```python
from build123d import *

# Parameters (mm, degrees)
SKETCH2_R          = 4.5
CUT_EXTRUDE1_DEPTH = 50


with BuildPart() as part:
    # Sketch1 → Base-Revolve (revolve)
    with BuildSketch(Plane.XY):
        with BuildLine():
            Line((0, 21), (0, 23.5))
            Line((0, 23.5), (0.5, 24))
            Line((0.5, 24), (5, 24))
            Line((5, 24), (5, 24.75))
            Line((5, 24.75), (13, 24.75))
            Line((13, 24.75), (13, 25))
            Line((13, 25), (2126.5, 25))
            Line((2126.5, 25), (2128, 24.133974596))
            Line((2128, 24.133974596), (2128, 23.8))
            ThreePointArc((2128, 23.8), (2128.234314575, 23.234314575), (2128.8, 23))
            Line((2128.8, 23), (2133.2, 23))
            ThreePointArc((2133.2, 23), (2133.765685425, 23.234314575), (2134, 23.8))
            Line((2134, 23.8), (2134, 24.25))
            ThreePointArc((2134, 24.25), (2134.146446609, 24.603553391), (2134.5, 24.75))
            Line((2134.5, 24.75), (2135.5, 24.75))
            Line((2135.5, 24.75), (2137, 23.883974596))
            Line((2137, 23.883974596), (2137, 23.55))
            ThreePointArc((2137, 23.55), (2137.234314575, 22.984314575), (2137.8, 22.75))
            Line((2137.8, 22.75), (2140, 22.75))
            Line((2140, 22.75), (2142.453263132, 24))
            Line((2142.453263132, 24), (2166.401923789, 24))
            Line((2166.401923789, 24), (2169, 22.5))
            Line((2169, 22.5), (2179, 22.5))
            Line((2179, 22.5), (2180, 21.922649731))
            Line((2180, 21.922649731), (2180, 17))
            Line((2180, 17), (6.92820323, 17))
            Line((6.92820323, 17), (0, 21))
        make_face()
    revolve(axis=Axis((0, 0, 0), (1, 0, 0)))

    # Sketch2 → Cut-Extrude1 (cut, symmetric)
    with BuildSketch(Plane.XY):
        with Locations((2116, 0)):
            Circle(SKETCH2_R)
    extrude(amount=CUT_EXTRUDE1_DEPTH, both=True, mode=Mode.SUBTRACT)


solid = part.part
```
CAD build for the part. Positions are in the model's coordinates, mm. A direction names the side the tool comes from. Coordinates: 2 decimals unless noted, no trailing zeros. Write each loop counter-clockwise with the first axis right and the second up, starting at its lowest first coordinate (ties: lowest second). Pieces come first, ordered by that corner, then holes. Notation, with made-up numbers: (76, 31) -> (122, 31) arc R29 ccw to (122, 56) -> close; hole circle Ø8 at (-34.5, -20). An arc over 180 degrees is marked (long way). Return JSON: item names as keys, results as strings. Group by question number.
Q1. Flat gauge pins, fed straight in: pin 1 (14.5 mm diameter, centred on y = -5.5, z = 11.5, fed in from -X); pin 2 (8 mm diameter, centred on x = 1127.5, y = 5, fed in from +Z); pin 3 (5 mm diameter, centred on x = 391, y = -1.5, fed in from -Z). Where does each tip first touch, or does it go through?
Q2. Which spindle directions (+Z, -Z, +X, -X, +Y, -Y) get a long thin tool onto all of the face, cutting with end or side? Do faces 4 (the face through (2174.07, 10.382, -19.961)), 5 (the face through (2131.031, -2.994, 22.804)), 6 (the face through (0, 18, -12)). Say none if no direction does.
Q3. Pull direction Z, two halves, no side cores. Call faces 1 (the face through (2135.01, -3.22, 24.54)), 2 (the face through (2137, 11, -21)), 3 (the face through (1078.253, 9.139, 14.334)): released by +Z, released by -Z, zero draft, split by the parting line, or undercut.
Q4. Drill centre lines: line 1 (X direction, y = 0, z = -21.25); line 2 (X direction, y = 16, z = -17.5); line 3 (Y direction, x = 1026.5, z = -4). Where is each one in solid material? Low to high.
Q5. Cut at A-A, the plane x = 1701. Give the cut face in (y, z).
Returned:
{
 "1": {"pin 1": "stops at x = 1.74", "pin 2": "stops at z = 24.98", "pin 3": "stops at z = -25"},
 "2": {"face 4": "+X", "face 5": "none", "face 6": "+Z, -Z, -X, +Y, -Y"},
 "3": {"face 1": "split by the parting line", "face 2": "zero draft", "face 3": "undercut"},
 "4": {"line 1": "x = 0 to 2111.5, 2120.5 to 2180", "line 2": "x = 0.21 to 2128, 2134 to 2137, 2141.89 to 2166.9", "line 3": "y = -24.68 to -16.52, 16.52 to 24.68"},
 "5": {"outline": "circle Ø50 at (0, 0); hole circle Ø34 at (0, 0)"}
}
